```python
from build123d import *

# Parameters (mm, degrees)
F0_R     = 1.75
F0_R_2   = 1.525
F0_R_3   = 7
F1_DEPTH = 2
F2_R     = 7.5
F3_DEPTH = 25


with BuildPart() as f1:
    # F0 (on Top) → F1 (new body)
    with BuildSketch(Plane.XY):
        with BuildLine():
            Line((-27.856726, 33.817827), (-28.563655, 34.41101))
            Line((-28.563655, 34.41101), (-38.848256, 22.154299))
            Line((-38.848256, 22.154299), (-21.575153, 7.660444))
            ThreePointArc((-21.575153, 7.660444), (-18.003029, 0), (-21.575153, -7.660444))
            Line((-21.575153, -7.660444), (-38.848256, -22.154299))
            Line((-38.848256, -22.154299), (-28.563655, -34.41101))
            Line((-28.563655, -34.41101), (-27.856726, -33.817827))
            ThreePointArc((-27.856726, -33.817827), (-21.46429, -32.976246), (-18, -38.414093))
            Line((-18, -38.414093), (-18, -69))
            ThreePointArc((-18, -69), (-16.535534, -72.535534), (-13, -74))
            Line((-13, -74), (0, -74))
            Line((0, -74), (13, -74))
            ThreePointArc((13, -74), (16.535534, -72.535534), (18, -69))
            Line((18, -69), (18, -38.414093))
            ThreePointArc((18, -38.414093), (21.46429, -32.976246), (27.856726, -33.817827))
            Line((27.856726, -33.817827), (28.563655, -34.41101))
            Line((28.563655, -34.41101), (38.848256, -22.154299))
            Line((38.848256, -22.154299), (21.575153, -7.660444))
            ThreePointArc((21.575153, -7.660444), (18.003029, 0), (21.575153, 7.660444))
            Line((21.575153, 7.660444), (38.848256, 22.154299))
            Line((38.848256, 22.154299), (28.563655, 34.41101))
            Line((28.563655, 34.41101), (27.856726, 33.817827))
            ThreePointArc((27.856726, 33.817827), (21.46429, 32.976246), (18, 38.414093))
            Line((18, 38.414093), (18, 69))
            ThreePointArc((18, 69), (16.535534, 72.535534), (13, 74))
            Line((13, 74), (0, 74))
            Line((0, 74), (-13, 74))
            ThreePointArc((-13, 74), (-16.535534, 72.535534), (-18, 69))
            Line((-18, 69), (-18, 38.414093))
            ThreePointArc((-18, 38.414093), (-21.46429, 32.976246), (-27.856726, 33.817827))
        make_face()
        with Locations((-13, -69)):
            Circle(F0_R, mode=Mode.SUBTRACT)
        with Locations((-28, -29)):
            Circle(F0_R_2, mode=Mode.SUBTRACT)
        with Locations((-28, -18)):
            Circle(F0_R_2, mode=Mode.SUBTRACT)
        with Locations((-14, -30)):
            Circle(F0_R_2, mode=Mode.SUBTRACT)
        with Locations((-15.25, -15.25)):
            Circle(F0_R_2, mode=Mode.SUBTRACT)
        with Locations((13, -69)):
            Circle(F0_R, mode=Mode.SUBTRACT)
        with Locations((14, -30)):
            Circle(F0_R_2, mode=Mode.SUBTRACT)
        with Locations((15.25, -15.25)):
            Circle(F0_R_2, mode=Mode.SUBTRACT)
        with Locations((28, -29)):
            Circle(F0_R_2, mode=Mode.SUBTRACT)
        with Locations((28, -18)):
            Circle(F0_R_2, mode=Mode.SUBTRACT)
        with Locations((-28, 18)):
            Circle(F0_R_2, mode=Mode.SUBTRACT)
        with Locations((-28, 29)):
            Circle(F0_R_2, mode=Mode.SUBTRACT)
        with Locations((-15.25, 15.25)):
            Circle(F0_R_2, mode=Mode.SUBTRACT)
        with Locations((-14, 30)):
            Circle(F0_R_2, mode=Mode.SUBTRACT)
        with Locations((-13, 69)):
            Circle(F0_R_2, mode=Mode.SUBTRACT)
        Circle(F0_R_3, mode=Mode.SUBTRACT)
        with Locations((15.25, 15.25)):
            Circle(F0_R_2, mode=Mode.SUBTRACT)
        with Locations((14, 30)):
            Circle(F0_R_2, mode=Mode.SUBTRACT)
        with Locations((28, 18)):
            Circle(F0_R_2, mode=Mode.SUBTRACT)
        with Locations((28, 29)):
            Circle(F0_R_2, mode=Mode.SUBTRACT)
        with Locations((13, 69)):
            Circle(F0_R_2, mode=Mode.SUBTRACT)
    extrude(amount=F1_DEPTH)

    # F2 (on face) → F3 (cut)
    with BuildSketch(Plane.XY.offset(2)):
        with Locations((0, -22)):
            Circle(F2_R)
        with Locations((0, 22)):
            Circle(F2_R)
        with BuildLine():
            ThreePointArc((-7.45, -44), (-9, -42.45), (-10.55, -44))
            Line((-10.55, -44), (-10.55, -60))
            ThreePointArc((-10.55, -60), (-9, -61.55), (-7.45, -60))
            Line((-7.45, -60), (-7.45, -44))
        make_face()
        with BuildLine():
            ThreePointArc((1.55, -44), (0, -42.45), (-1.55, -44))
            Line((-1.55, -44), (-1.55, -60))
            ThreePointArc((-1.55, -60), (0, -61.55), (1.55, -60))
            Line((1.55, -60), (1.55, -44))
        make_face()
        with BuildLine():
            ThreePointArc((10.55, -44), (9, -42.45), (7.45, -44))
            Line((7.45, -44), (7.45, -60))
            ThreePointArc((7.45, -60), (9, -61.55), (10.55, -60))
            Line((10.55, -60), (10.55, -44))
        make_face()
        with BuildLine():
            ThreePointArc((-9, 62), (-10, 63), (-11, 62))
            Line((-11, 62), (-11, 38))
            ThreePointArc((-11, 38), (-10, 37), (-9, 38))
            Line((-9, 38), (-9, 62))
        make_face()
        with BuildLine():
            ThreePointArc((-4, 62), (-5, 63), (-6, 62))
            Line((-6, 62), (-6, 38))
            ThreePointArc((-6, 38), (-5, 37), (-4, 38))
            Line((-4, 38), (-4, 62))
        make_face()
        with BuildLine():
            ThreePointArc((1, 62), (0, 63), (-1, 62))
            Line((-1, 62), (-1, 38))
            ThreePointArc((-1, 38), (0, 37), (1, 38))
            Line((1, 38), (1, 62))
        make_face()
        with BuildLine():
            ThreePointArc((6, 62), (5, 63), (4, 62))
            Line((4, 62), (4, 38))
            ThreePointArc((4, 38), (5, 37), (6, 38))
            Line((6, 38), (6, 62))
        make_face()
        with BuildLine():
            ThreePointArc((11, 62), (10, 63), (9, 62))
            Line((9, 62), (9, 38))
            ThreePointArc((9, 38), (10, 37), (11, 38))
            Line((11, 38), (11, 62))
        make_face()
    extrude(amount=-F3_DEPTH, mode=Mode.SUBTRACT)


solid = f1.part
```
The model under review builds one solid part; all positions refer to its coordinate system, in mm. A direction names the side the tool comes from. Give positions to 0.01 mm unless a question says otherwise; leave off trailing zeros. Write each loop counter-clockwise with the first axis right and the second up, starting at its lowest first coordinate (ties: lowest second). Pieces come first, ordered by that corner, then holes.
(1) To check wall thickness, follow L1, parallel to X at y = 57.5, z = 1.05; L2, parallel to X at y = -45.5, z = 0.5; L3, parallel to X at y = 69, z = 1.4 (3 decimals). State the ranges of each line that lie inside material, in increasing order.
(2) The part is to be moulded in two halves that separate along X. For faces 4 (the flat face through (-33.634, 28.368, 0.986)), 5 (the cylindrical face through (-29.21, 17.07, 0.99)), 6 (the cylindrical face through (18.004, -0.122, 0.986)), say which applies: released by +X, released by -X, zero draft, split by the parting line, or undercut.
(3) Consider section B-B, the plane x = -33. Give the boundary of the cut face in (y, z), and give its area (3 significant figures).
(4) Consider section C-C, the plane y = 57. Give the boundary of the cut face in (x, z).
(5) Consider section D-D, the plane z = 1.35. Give the number of separate pieces and of enclosed holes in the cut face, and give its area (3 significant figures).
(6) Consider section A-A, the plane y = 0. Give the boundary of the cut face in (x, z).
(7) Tool access review of faces 1 (the flat face through (30.333, -15.009, 0.986)), 2 (the cylindrical face through (-13.2, 70.51, 0.99)), 3 (the flat face through (-30.091, -14.806, 0.986)): name each direction out of +Z, -Z, +X, -X, +Y, -Y from which nothing blocks a thin tool from reaching the whole face with its end or side.
(8) For P1, Ø0.6, axis at y = 53.5, z = 1, coming from the +X side; P2, Ø2.5, axis at x = 14, y = -30, coming from the -Z side; P3, Ø1, axis at y = 48.5, z = 1, coming from the -X side, all flat-tipped, find the tip position at first contact; note any pin that passes through.
Returned:
1. L1: x = -18 to -11, -9 to -6, -4 to -1, 1 to 4, 6 to 9, 11 to 18
1. L2: x = -18 to -10.55, -7.45 to -1.55, 1.55 to 7.45, 10.55 to 18
1. L3: x = -18 to -14.525, -11.475 to 11.475, 14.525 to 18
2. face 4: released by -X
2. face 5: undercut
2. face 6: released by +X
3. outline: (-29.12, 0) - (-17.25, 0) - (-17.25, 2) - (-29.12, 2) - close; (17.25, 0) - (29.12, 0) - (29.12, 2) - (17.25, 2) - close
3. area: 47.5 mm2
4. outline: (-18, 0) - (-11, 0) - (-11, 2) - (-18, 2) - close; (-9, 0) - (-6, 0) - (-6, 2) - (-9, 2) - close; (-4, 0) - (-1, 0) - (-1, 2) - (-4, 2) - close; (1, 0) - (4, 0) - (4, 2) - (1, 2) - close; (6, 0) - (9, 0) - (9, 2) - (6, 2) - close; (11, 0) - (18, 0) - (18, 2) - (11, 2) - close
5. separate pieces: 1
5. enclosed holes: 31
5. area: 5,690 mm2
6. outline: (-18, 0) - (-7, 0) - (-7, 2) - (-18, 2) - close; (7, 0) - (18, 0) - (18, 2) - (7, 2) - close
7. face 1: +Z, -Z, +X
7. face 2: +Z, -Z
7. face 3: +Z, -Z, -X
8. P1: stops at x = 18
8. P2: passes through
8. P3: stops at x = -18
